Read the model definition and answer for the solid it produces. Units are mm, in the model's axes. A direction names the side the tool comes from. Coordinates: 2 decimals unless noted, no trailing zeros. Loops run counter-clockwise (first coordinate to the right, second up) from the corner with the lowest first, then second, coordinate; pieces in that order, holes last. Notation, with made-up numbers: M 25.5,41 L 46.5,41 A8 cw 46.5,49 Z; hole C -15,-21 d1. An arc over 180 degrees is marked long. One line per item, written item: value. Start each with the question number.
1. Flat-ended cylindrical pins translate along their axes: pin 1 (5 mm diameter, centred on x = 39, y = -70.5, fed in from -Z); pin 2 (12 mm diameter, centred on x = 95, z = -28, fed in from -Y); pin 3 (5 mm diameter, centred on x = 48, y = -48.5, fed in from +Z). Find the tip coordinate at first contact, or state that the pin passes through.
2. The part is cut by section B-B (x = 0). Write down the section's boundary in (y, z) (3 decimals), then the cut area to 3 significant figures.
3. The part is cut by section C-C (z = 3.5). Write down the section's boundary in (x, y) (3 decimals), then the cut area to 3 significant figures.
4. Determine the mould class of faces 4 (the face through (-40, -69, -16)), 5 (the face through (103, -44, 28)), 6 (the face through (70.01, -33, 0)), 7 (the face through (-6.194, -31.552, 27.895)) for opening direction Z: +Z half, -Z half, draft (parallel to the pull), parting line (faces both ways), or undercut.
5. Consider probe 1 along Z at (x, y) = (108, -37); probe 2 along X at (y, z) = (-63, -1.5); probe 3 along Z at (x, y) = (0, -36) (3 decimals). Determine where each line is inside the solid, lowest interval first.
6. The part is cut by section D-D (y = -52). Write down the section's boundary in (x, z) (3 decimals), then the cut area to 3 significant figures.
7. For faces 1 (the face through (40, -69, -16.621)), 2 (the face through (126, -33, 25)), 3 (the face through (109, -22, -41)), determine the directions among +Z, -Z, +X, -X, +Y, -Y from which every point of the face is accessible in a straight line to the end or side of a thin tool.
8. The part is cut by section A-A (y = -13). Write down the section's boundary in (x, z) (3 decimals).
```python
from build123d import *

# Parameters (mm, degrees)
F0_R     = 11.1
F1_DEPTH = 22
F2_DEPTH = 44
F3_DEPTH = 64
F4_DEPTH = 74
F5_SIZE  = 12


with BuildPart() as f1:
    # F0 (on Front) → F1 (new body)
    with BuildSketch(Plane.XZ):
        Polygon((184.0099021196, -25), (184.0099021196, 25), (70.0099021196, 25), (70.0099021196, 0), (70.0099021196, -25), align=None)
        with Locations((99.0099021196, 0)):
            Circle(F0_R, mode=Mode.SUBTRACT)
        with Locations((149.0099021196, 0)):
            Circle(F0_R, mode=Mode.SUBTRACT)
    extrude(amount=F1_DEPTH)

    # F0 (on Front) → F2 (join)
    with BuildSketch(Plane.XZ):
        with BuildLine():
            ThreePointArc((51.5751878329, 16), (53.3903556037, 8.0913489921), (54, 0))
            ThreePointArc((54, 0), (53.9991081797, -0.3103478577), (53.9964327484, -0.6206854644))
            ThreePointArc((53.9964327484, -0.6206854644), (53.2913728634, -8.7194941557), (51.3785248396, -16.6206854644))
            ThreePointArc((51.3785248396, -16.6206854644), (44.9451061645, -29.9322139486), (35.1425667816, -41))
            Line((35.1425667816, -41), (184.0099021196, -41))
            Line((184.0099021196, -41), (184.0099021196, -25))
            Line((184.0099021196, -25), (70.0099021196, -25))
            Line((70.0099021196, -25), (70.0099021196, 0))
            Line((70.0099021196, 0), (70.0099021196, 25))
            Line((70.0099021196, 25), (184.0099021196, 25))
            Line((184.0099021196, 25), (184.0099021196, 41))
            Line((184.0099021196, 41), (35.1425667816, 41))
            ThreePointArc((35.1425667816, 41), (45.1247409006, 29.6607106903), (51.5751878329, 16))
        make_face()
    extrude(amount=F2_DEPTH)

    # F0 (on Front) → F3 (join)
    with BuildSketch(Plane.XZ):
        with BuildLine():
            Line((28.575, 16), (51.5751878329, 16))
            ThreePointArc((51.5751878329, 16), (45.1247409006, 29.6607106903), (35.1425667816, 41))
            ThreePointArc((35.1425667816, 41), (-14.9585346426, 51.8868214612), (-51.5751878329, 16))
            Line((-51.5751878329, 16), (-28.575, 16))
            Line((-28.575, 16), (-28.575, 0))
            ThreePointArc((-28.575, 0), (0, 28.575), (28.575, 0))
            Line((28.575, 0), (28.575, 16))
        make_face()
        with BuildLine():
            ThreePointArc((35.1425667816, -41), (44.9451061645, -29.9322139486), (51.3785248396, -16.6206854644))
            Line((51.3785248396, -16.6206854644), (28.575, -16.6206854644))
            Line((28.575, -16.6206854644), (28.575, -0.6206854644))
            Line((28.575, -0.6206854644), (28.575, 0))
            ThreePointArc((28.575, 0), (0, -28.575), (-28.575, 0))
            Line((-28.575, 0), (-28.575, -16))
            Line((-28.575, -16), (-51.5751878329, -16))
            ThreePointArc((-51.5751878329, -16), (-14.9585346426, -51.8868214612), (35.1425667816, -41))
        make_face()
    extrude(amount=F3_DEPTH)

    # F0 (on Front) → F4 (join)
    with BuildSketch(Plane.XZ):
        with BuildLine():
            ThreePointArc((53.9964327484, -0.6206854644), (53.9991081797, -0.3103478577), (54, 0))
            ThreePointArc((54, 0), (53.3903556037, 8.0913489921), (51.5751878329, 16))
            Line((51.5751878329, 16), (28.575, 16))
            Line((28.575, 16), (28.575, 0))
            Line((28.575, 0), (28.575, -0.6206854644))
            Line((28.575, -0.6206854644), (28.575, -16.6206854644))
            Line((28.575, -16.6206854644), (51.3785248396, -16.6206854644))
            ThreePointArc((51.3785248396, -16.6206854644), (53.2913728634, -8.7194941557), (53.9964327484, -0.6206854644))
        make_face()
        with BuildLine():
            Line((-28.575, 16), (-51.5751878329, 16))
            ThreePointArc((-51.5751878329, 16), (-54, 0), (-51.5751878329, -16))
            Line((-51.5751878329, -16), (-28.575, -16))
            Line((-28.575, -16), (-28.575, 0))
            Line((-28.575, 0), (-28.575, 16))
        make_face()
    extrude(amount=F4_DEPTH)

    # F5
    f5_edges = [f1.edges().sort_by_distance(p)[0] for p in [
        (184.009902, -44, 33),
        (184.009902, -44, -33),
    ]]
    chamfer(f5_edges, length=F5_SIZE)


solid = f1.part
```
Answer block:
1. pin 1: stops at z = -16.62
1. pin 2: stops at y = -44
1. pin 3: stops at z = 29.08
2. outline: M -64,-54 L 0,-54 L 0,-28.575 L -64,-28.575 Z; M -64,28.575 L 0,28.575 L 0,54 L -64,54 Z
2. area: 3,250 mm2
3. outline: M -53.886,-74 L -28.575,-74 L -28.575,-64 L -28.36,-64 L -28.36,0 L -53.886,0 Z; M 28.36,-64 L 28.575,-64 L 28.575,-74 L 53.886,-74 L 53.886,-44 L 70.01,-44 L 70.01,-22 L 88.476,-22 L 88.476,0 L 28.36,0 Z; M 109.544,-22 L 138.476,-22 L 138.476,0 L 109.544,0 Z; M 159.544,-22 L 184.01,-22 L 184.01,0 L 159.544,0 Z
3. area: 6,060 mm2
4. face 4: -Z half
4. face 5: draft
4. face 6: undercut
4. face 7: undercut
5. probe 1: z = -41 to -25, 25 to 41
5. probe 2: x = -53.98 to -28.54, 28.54 to 53.98
5. probe 3: z = -54 to -28.575, 28.575 to 54
6. outline: M 53.996,-0.621 A54 ccw 54,0 A54 ccw long Z; hole C 0,0 d57.15
6. area: 6,600 mm2
7. face 1: -Z, +X, -X, -Y
7. face 2: +X, -Y
7. face 3: -Z, +X, +Y, -Y
8. outline: M 35.143,-41 L 184.01,-41 L 184.01,41 L 35.143,41 A54 ccw long Z; hole C 0,0 d57.15; hole C 99.01,0 d22.2; hole C 149.01,0 d22.2
